For this review, take the finished solid that the model builds, in its own axes (mm). Face numbers are marked on the shaded views. A direction names the side the tool comes from. Round coordinates to 2 decimals unless told otherwise and drop trailing zeros. Order: outer loops, then holes, each group sorted by start corner. A loop starts at its lowest first (then second) coordinate and runs counter-clockwise, first axis right, second up. Notation, with made-up numbers: M -9.75,75.25 L 24.25,75.25 A16 ccw 24.25,94.25 Z; hole C 29,47.25 d10. An arc over 180 degrees is marked long. Put each result on its own line as item: value.
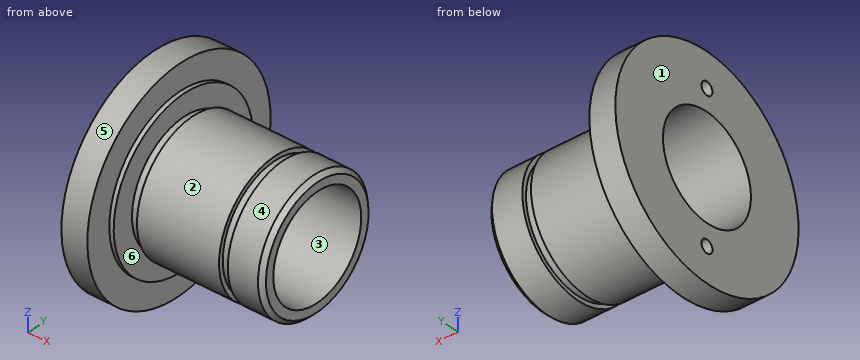
from build123d import *

# Parameters (mm, degrees)
F2_SIZE  = 1
F4_D     = 3
F4_DEPTH = 5
F4_TIP   = 0.9012909285


with BuildPart() as f1:
    # F0 (on Front) → F1 (revolve)
    with BuildSketch(Plane.XZ):
        Polygon((0, 25), (0, 12), (38, 12), (38, 15), (30, 15), (30, 14), (28, 14), (28, 15), (9, 15), (9, 14), (7, 14), (7, 19), (6, 19), (6, 25), align=None)
    revolve(axis=Axis((16.4548096063, 0, 0), (1, 0, 0)))

    # F2
    f2_edges = [f1.edges().sort_by_distance(p)[0] for p in [
        (38, 0, -15),
    ]]
    chamfer(f2_edges, length=F2_SIZE)

    # F4
    with Locations(Plane(origin=(0, 0, 0), x_dir=(0, -1, 0), z_dir=(-1, 0, 0))):
        with Locations((0, 17), (0, -17)):
            Hole(F4_D / 2, depth=F4_DEPTH)
            with Locations((0, 0, -(F4_DEPTH + F4_TIP / 2))):  # 118° drill point
                Cone(0, F4_D / 2, F4_TIP, mode=Mode.SUBTRACT)


solid = f1.part
(1) To check wall thickness, follow L1, parallel to Z at x = 3.9, y = 0; L2, parallel to Y at x = 24.5, z = 0; L3, parallel to X at y = -19, z = 14. State the ranges of each line that lie inside material, in increasing order.
A:
L1: z = -25 to -18.5, -15.5 to -12, 12 to 15.5, 18.5 to 25
L2: y = -15 to -12, 12 to 15
L3: x = 0 to 6
(2) Draft analysis for pull direction Y (two halves, no side actions). For the marked faces 1, 2 and 3, state which applies: released by +Y, released by -Y, zero draft, split by the parting line, or undercut.
A:
face 1: zero draft
face 2: split by the parting line
face 3: undercut
(3) Add section D-D on y = -21.5. Give the boundary of the cut face in (x, z).
A:
outline: M 0,-12.76 L 6,-12.76 L 6,12.76 L 0,12.76 Z
(4) Add section C-C on x = 32. Give the boundary of the cut face in (y, z), then the cut area to 3 significant figures.
A:
outline: C 0,0 d30; hole C 0,0 d24
area: 254 mm2
(5) Add section B-B on y = 16.5. Give the boundary of the cut face in (x, z).
A:
outline: M 0,-18.78 L 6,-18.78 L 6,-9.42 L 7,-9.42 L 7,9.42 L 6,9.42 L 6,18.78 L 0,18.78 Z
(6) For the marked faces 4, 5 and 6, list the 3-axis set-ups (+Z, -Z, +X, -X, +Y, -Y) from which the entire face can be reached by the end or side of a thin tool; tool diameter is ignored.
A:
face 4: +X
face 5: +X, -X
face 6: none
(7) Insertion check: pin 1 Ø1.5 at (x, y) = (33.5, 13.5) entering from -Z; pin 2 Ø4 at (x, z) = (25.5, -0.5) entering from -Y; pin 3 Ø10 at (x, z) = (7, -4) entering from -Y. Each pin has a flat end and moves straight along its axis. Give the tip position at first contact, or say it passes through.
A:
pin 1: stops at z = -7.9
pin 2: stops at y = -15
pin 3: stops at y = -25
